from build123d import *

# Parameters (mm, degrees)
SKETCH3_W           = 25.7
SKETCH3_H           = 39.2
SKETCH3_W_2         = 14.4
SKETCH3_H_2         = 29.9
BOSS_EXTRUDE2_DEPTH = 12
CHAMFER1_SIZE       = 1
CHAMFER1_SIZE2      = 10
SKETCH4_W           = 20.4
SKETCH4_H           = 35.9
SKETCH4_W_2         = 14.4
SKETCH4_H_2         = 29.9


with BuildPart() as part:
    # Sketch3 → Boss-Extrude2 (new body)
    with BuildSketch(Plane.XY):
        with Locations((12.85, 19.6)):
            Rectangle(SKETCH3_W, SKETCH3_H)
        with Locations((12.85, 19.6)):
            Rectangle(SKETCH3_W_2, SKETCH3_H_2, mode=Mode.SUBTRACT)
    extrude(amount=BOSS_EXTRUDE2_DEPTH)

    # Chamfer1
    chamfer1_edges = [part.edges().sort_by_distance(p)[0] for p in [
        (5.65, 19.6, 0),
        (12.85, 4.65, 0),
        (20.05, 19.6, 0),
        (12.85, 34.55, 0),
        (12.85, 39.2, 0),
        (25.7, 19.6, 0),
        (12.85, 0, 0),
        (0, 19.6, 0),
    ]]
    chamfer1_side = [part.faces().sort_by_distance(p)[0] for p in [
        (12.85, 0.468735533, 0),
    ]]
    chamfer(chamfer1_edges, length=CHAMFER1_SIZE, length2=CHAMFER1_SIZE2, reference=chamfer1_side[0])

    # Sweep1: sweep along a path in Sketch6
    with BuildLine(Plane.ZY.offset(-12.85)) as sweep1_path:
        Line((12, 1.65), (24.024266767, -5.292213655))
    # Sketch4 → Sweep1 (sweep)
    with BuildSketch(Plane.XY.offset(12)):
        with Locations((12.85, 19.6)):
            Rectangle(SKETCH4_W, SKETCH4_H)
        with Locations((12.85, 19.6)):
            Rectangle(SKETCH4_W_2, SKETCH4_H_2, mode=Mode.SUBTRACT)
    sweep(path=sweep1_path.line)


solid = part.part
Verification items for the finished model (mm, model axes). A direction names the side the tool comes from. Coordinates: 2 decimals unless noted, no trailing zeros. Loops run counter-clockwise (first coordinate to the right, second up) from the corner with the lowest first, then second, coordinate; pieces in that order, holes last. Notation, with made-up numbers: (68.5, 82.5) -> (104.5, 82.5) arc R16 cw to (104.5, 97.5) -> close; hole circle Ø6 at (-19, 54.25). An arc over 180 degrees is marked (long way). Write each question's results on one line, items separated by ' | '.
Item 1: Material ranges on L1, parallel to X at y = 12.5, z = 18.25; L2, parallel to X at y = 26, z = 10.5; L3, parallel to Y at x = 11, z = 10.5, recorded low to high.
Found:
L1: x = 2.65 to 5.65, 20.05 to 23.05 | L2: x = 0 to 5.65, 20.05 to 25.7 | L3: y = 0 to 4.65, 34.55 to 39.2
Item 2: Tool access check on faces 1 (the face through (5.65, 16, 17)), 2 (the face through (12.95, 1.13, 18.1)), 3 (the face through (2.65, 16, 18)), 4 (the face through (13, 34.55, 11)). Record the directions out of +Z, -Z, +X, -X, +Y, -Y that give a thin tool (end or side, any length) a straight path to the whole face; none if there is none.
Found:
face 1: none | face 2: +Z | face 3: +Z, -X, +Y, -Y | face 4: -Z
Item 3: Mould release check, pull along Y, two halves, no side actions. Record for faces 5 (the face through (0, 19, 11)), 6 (the face through (13, 0, 11)), 7 (the face through (5.157, 19.377, 5.07)): +Y half, -Y half, draft (parallel to the pull), parting line (faces both ways), or undercut.
Found:
face 5: draft | face 6: -Y half | face 7: undercut
Item 4: Section check C-C, the plane y = 21. Enter the section's corners in (x, z).
Found:
outline: (0, 10) -> (1, 0) -> (4.65, 0) -> (5.65, 10) -> (5.65, 24.02) -> (2.65, 24.02) -> (2.65, 12) -> (0, 12) -> close; (20.05, 10) -> (21.05, 0) -> (24.7, 0) -> (25.7, 10) -> (25.7, 12) -> (23.05, 12) -> (23.05, 24.02) -> (20.05, 24.02) -> close
Item 5: Gauge pin test, flat ends, axial feed: pin 1 (13 mm diameter, centred on x = 11.5, y = 10.5, fed in from +Z); pin 2 (3 mm diameter, centred on x = 6, z = 14, fed in from -Y); pin 3 (0.6 mm diameter, centred on x = 15.5, z = 11, fed in from -Y); pin 4 (10 mm diameter, centred on y = 19, z = 21.5, fed in from -X). Record the tip position at first contact, or that the pin passes through.
Found:
pin 1: stops at z = 24.02 | pin 2: stops at y = -0.37 | pin 3: stops at y = 0 | pin 4: stops at x = 2.65
Item 6: Section check D-D, the plane z = 1.5. Enter the section's corners in (x, y), plus the area to 3 significant figures.
Found:
outline: (0.85, 0.85) -> (24.85, 0.85) -> (24.85, 38.35) -> (0.85, 38.35) -> close; hole (4.8, 3.8) -> (20.9, 3.8) -> (20.9, 35.4) -> (4.8, 35.4) -> close | area: 391 mm2
Item 7: Section check B-B, the plane z = 11. Enter the section's corners in (x, y), plus the area to 3 significant figures.
Found:
outline: (0, 0) -> (25.7, 0) -> (25.7, 39.2) -> (0, 39.2) -> close; hole (5.65, 4.65) -> (20.05, 4.65) -> (20.05, 34.55) -> (5.65, 34.55) -> close | area: 577 mm2
Item 8: Section check A-A, the plane x = 9. Enter the section's corners in (y, z), plus the area to 3 significant figures.
Found:
outline: (-5.29, 24.02) -> (1.65, 12) -> (0, 12) -> (0, 10) -> (1, 0) -> (3.65, 0) -> (4.65, 10) -> (4.65, 12) -> (-2.29, 24.02) -> close; (27.61, 24.02) -> (34.55, 12) -> (34.55, 10) -> (35.55, 0) -> (38.2, 0) -> (39.2, 10) -> (39.2, 12) -> (37.55, 12) -> (30.61, 24.02) -> close | area: 164 mm2
